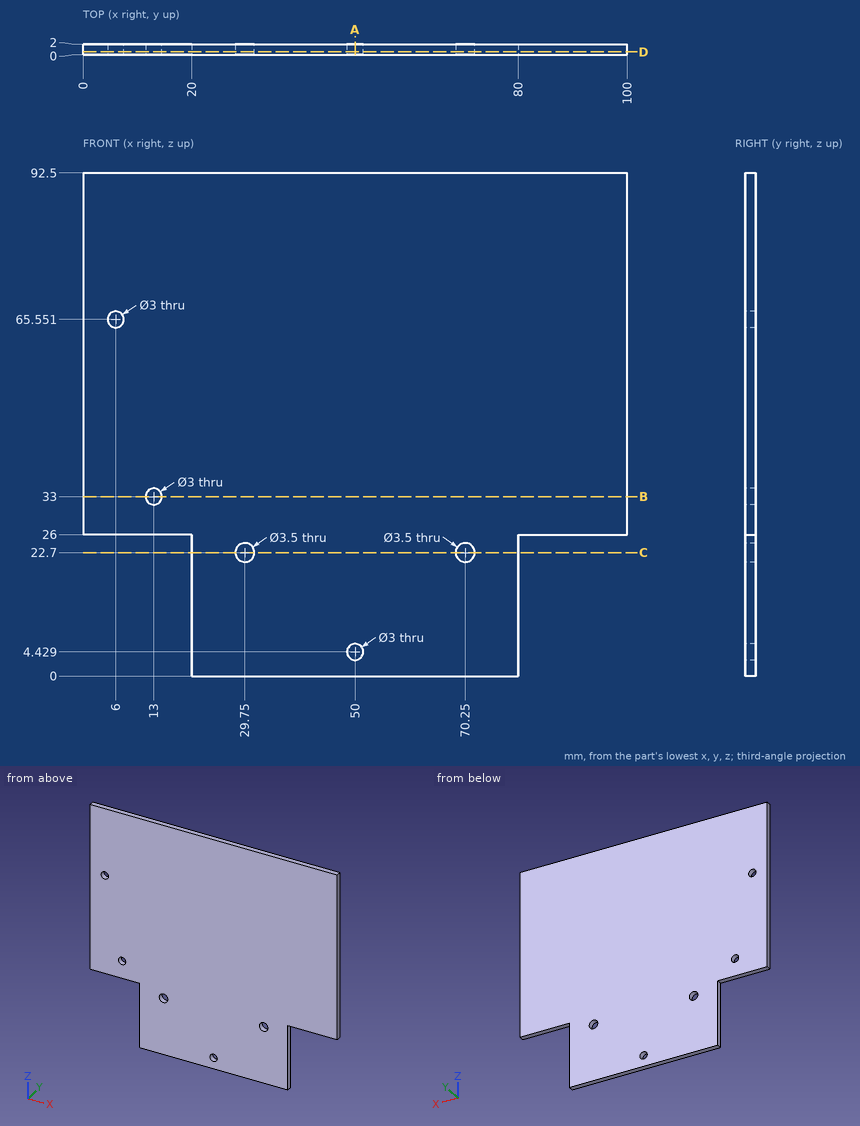
Part print with two shaded views. Sizes in mm from the minimum x, y, z corner. Round coordinates to 2 decimals unless told otherwise and drop trailing zeros. Order: outer loops, then holes, each group sorted by start corner. A loop starts at its lowest first (then second) coordinate and runs counter-clockwise, first axis right, second up. Notation, with made-up numbers: M -8.75,82.25 L 45.25,82.25 A16 ccw 45.25,106.25 Z; hole C 46,84 d5. An arc over 180 degrees is marked long. Use CSV: the item, a comma, the result in double quotes.
Item 1: Saw through at B-B (z = 33). List the corners of the cut face in (x, y).
Worked answers:
outline,"M 0,0 L 11.5,0 L 11.5,2 L 0,2 Z; M 14.5,0 L 100,0 L 100,2 L 14.5,2 Z"
Item 2: Saw through at D-D (y = 0.55). List the corners of the cut face in (x, z), plus the area to 3 significant figures.
Worked answers:
outline,"M 0,26 L 20,26 L 20,0 L 80,0 L 80,26 L 100,26 L 100,92.5 L 0,92.5 Z; hole C 6,65.55 d3; hole C 13,33 d3; hole C 29.75,22.7 d3.5; hole C 50,4.43 d3; hole C 70.25,22.7 d3.5"
area,"8,170 mm²"
Item 3: Pin check, flat tips, straight feed: pin 1 (0.6 mm diameter, centred on x = 5, y = 0.5, fed in from -Z); pin 2 (0.6 mm diameter, centred on y = 1, z = 8.5, fed in from -X); pin 3 (1 mm diameter, centred on y = 0.5, z = 6.5, fed in from +X). Stop position of each tip, or through.
Worked answers:
pin 1,"z = 26"
pin 2,"x = 20"
pin 3,"x = 80"
Item 4: Saw through at A-A (x = 50). List the corners of the cut face in (y, z).
Worked answers:
outline,"M 0,0 L 2,0 L 2,2.93 L 0,2.93 Z; M 0,5.93 L 2,5.93 L 2,92.5 L 0,92.5 Z"
Item 5: Saw through at C-C (z = 22.7). List the corners of the cut face in (x, y).
Worked answers:
outline,"M 20,0 L 28,0 L 28,2 L 20,2 Z; M 31.5,0 L 68.5,0 L 68.5,2 L 31.5,2 Z; M 72,0 L 80,0 L 80,2 L 72,2 Z"
Item 6: Probe probe 1 along Z at (x, y) = (70.25, 1.2); probe 2 along X at (y, z) = (0.4, 23.5); probe 3 along Z at (x, y) = (6, 0.2). List the from-to ranges inside material, lowest first.
Worked answers:
probe 1,"0 to 20.95, 24.45 to 92.5"
probe 2,"20 to 28.19, 31.31 to 68.69, 71.81 to 80"
probe 3,"26 to 64.05, 67.05 to 92.5"
